Build history of the part. All positions in model axes, mm. A direction names the side the tool comes from. Give positions to 0.01 mm unless a question says otherwise; leave off trailing zeros. Loops run counter-clockwise (first coordinate to the right, second up) from the corner with the lowest first, then second, coordinate; pieces in that order, holes last. Notation, with made-up numbers: (87.25, 0.25) - (127.25, 0.25) arc R26 ccw to (127.25, 26.25) - close; hole circle Ø3 at (54, 46). An arc over 180 degrees is marked (long way). Return JSON: item names as keys, results as strings. Group by question number.
1) Slice it at A-A (y = 23.5). List the corners of the cut face in (x, z).
2) 3-axis set-ups, long thin cutter, end or side, ignore diameter. For faces 5 (the face through (-20, 105, 16)), 6 (the face through (-25.5, 37, 21.1)), 7 (the face through (-20, 26, 31)): which of +Z, -Z, +X, -X, +Y, -Y reach the whole face in a straight line?
3) Slice it at C-C (z = 16). List the corners of the cut face in (x, y).
4) Mould opens along Z. For faces 1 (the face through (-20, 52, 0)), 2 (the face through (0, 52, 16)), 3 (the face through (-20, 75, 16)), 4 (the face through (-20, 23, 29)) say: released by +Z, released by -Z, zero draft, split by the parting line, or undercut.
5) Slice it at B-B (z = 11.5). List the corners of the cut face in (x, y), and give its area (3 significant figures).
6) Drop flat-ended pins along their axis: pin 1 (1 mm diameter, centred on x = -13, y = 74.5, fed in from -Z); pin 2 (4.5 mm diameter, centred on x = -18.5, z = 18, fed in from -Y). Give the stop position or say it passes through.
7) Drill centre lines: probe 1 along X at (y, z) = (53.5, 16); probe 2 along Z at (x, y) = (-20, 30.5); probe 3 along Z at (x, y) = (-20, 89). Where is each one in solid material? Low to high. Write a range as from..to.
8) Slice it at D-D (x = -25.5). List the corners of the cut face in (y, z).
```python
from build123d import *

# Parameters (mm, degrees)
F0_W     = 40
F0_H     = 32
F1_DEPTH = 105
F2_R     = 7.5
F3_DEPTH = 75
F4_R     = 3
F5_DEPTH = 105.001
F7_R     = 67.5
F8_DEPTH = 6


with BuildPart() as f1:
    # F0 (on Front) → F1 (new body)
    with BuildSketch(Plane.XZ):
        with Locations((-20, 16)):
            Rectangle(F0_W, F0_H)
    extrude(amount=-F1_DEPTH)

    # F2 (on face) → F3 (cut)
    with BuildSketch(Plane.XZ):
        with Locations((-20, 16)):
            Circle(F2_R)
    extrude(amount=-F3_DEPTH, mode=Mode.SUBTRACT)

    # F4 (on Front) → F5 (cut, through all)
    with BuildSketch(Plane.XZ):
        with Locations((-20, 11.5)):
            Circle(F4_R)
    extrude(amount=-F5_DEPTH, mode=Mode.SUBTRACT)

    # F7 (on offset) → F8 (cut)
    with BuildSketch(Plane.XZ.offset(-20)):
        with Locations((-20, 96.5)):
            Circle(F7_R)
    extrude(amount=-F8_DEPTH, mode=Mode.SUBTRACT)


solid = f1.part
```
Results:
{
 "1": {"outline": "(-40, 0) - (0, 0) - (0, 32) - (-0.1, 32) arc R67.5 cw to (-39.9, 32) - (-40, 32) - close; hole circle Ø15 at (-20, 16)"},
 "2": {"face 5": "+Z, -Z, +X, -X, +Y", "face 6": "-Y", "face 7": "+Z"},
 "3": {"outline": "(-40, 0) - (-27.5, 0) - (-27.5, 75) - (-12.5, 75) - (-12.5, 0) - (0, 0) - (0, 105) - (-40, 105) - close"},
 "4": {"face 1": "released by -Z", "face 2": "zero draft", "face 3": "undercut", "face 4": "released by +Z"},
 "5": {"outline": "(-40, 0) - (-26, 0) - (-26, 75) - (-23, 75) - (-23, 105) - (-40, 105) - close; (-17, 75) - (-14, 75) - (-14, 0) - (0, 0) - (0, 105) - (-17, 105) - close", "area": "3,120 mm2"},
 "6": {"pin 1": "z = 0", "pin 2": "y = 75"},
 "7": {"probe 1": "-40..-27.5, -12.5..0", "probe 2": "0..8.5, 23.5..32", "probe 3": "0..8.5, 14.5..32"},
 "8": {"outline": "(0, 0) - (105, 0) - (105, 32) - (26, 32) - (26, 29.22) - (20, 29.22) - (20, 32) - (0, 32) - (0, 21.1) - (75, 21.1) - (75, 10.9) - (0, 10.9) - close"}
}
